```python
from build123d import *

# Parameters (mm, degrees)
SKETCH_R     = 50
PAD_DEPTH    = 3
SKETCH001_R  = 16
POCKET_DEPTH = 3.001
FILLET_R     = 1.2


with BuildPart() as part:
    # Sketch → Pad (new body)
    with BuildSketch(Plane.XY):
        Circle(SKETCH_R)
    extrude(amount=PAD_DEPTH)

    # Sketch001 (on Face3 of Pad) → Pocket (cut, through all)
    with BuildSketch(Plane.XY.offset(3)):
        Circle(SKETCH001_R)
    extrude(amount=-POCKET_DEPTH, mode=Mode.SUBTRACT)

    # Fillet
    fillet_edges = [part.edges().sort_by_distance(p)[0] for p in [
        (-16, 0, 3),
        (16, 0, 1.5),
        (-16, 0, 0),
        (50, 0, 1.5),
        (-50, 0, 0),
        (-50, 0, 3),
    ]]
    fillet(fillet_edges, radius=FILLET_R)


solid = part.part
```
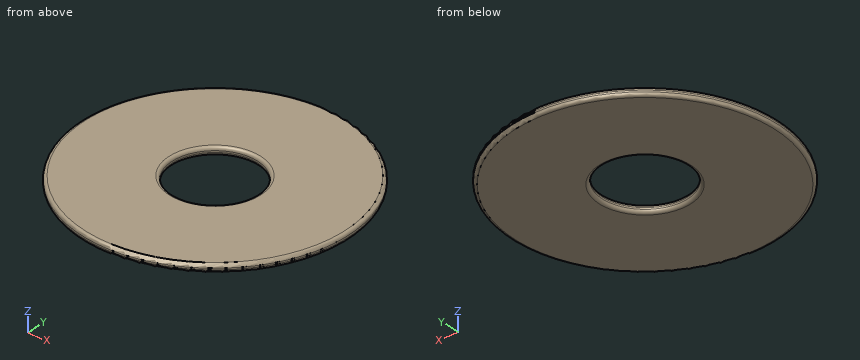
Geometry: final body of the model. Coordinates: model frame, mm. Coordinates: 2 decimals unless noted, no trailing zeros. Loops run counter-clockwise (first coordinate to the right, second up) from the corner with the lowest first, then second, coordinate; pieces in that order, holes last. Notation, with made-up numbers: (3, 67.25) -> (51, 67.25) arc R7 ccw to (51, 76.25) -> close; hole circle Ø3 at (-6.75, 73.5). An arc over 180 degrees is marked (long way). Use a Markdown table: item, result. Add a question column.
(1) Line query: line 1 along Y through (x, z) = (0, 1.6); line 2 along Y through (x, z) = (-3, 2.1); line 3 along X through (y, z) = (11, 0.8). Output: solid intervals per line, ascending.
(2) Section query A-A, the plane x = 0. Return loops of the section in (y, z).
(3) Pin query (flat end, axial travel): pin 1 Ø3 at (x, y) = (20.5, 26.5) entering from -Z; pin 2 Ø1.5 at (x, z) = (-12, 2.5) entering from -Y; pin 3 Ø1 at (x, z) = (32, 1.5) entering from +Y. Return the tip coordinate at first contact, or that it passes through.
(4) Section query C-C, the plane z = 2.4. Return loops of the section in (x, y).
Answer:
| question | item | result |
|---|---|---|
| 1 | line 1 | y = -50 to -16, 16 to 50 |
| 1 | line 2 | y = -49.87 to -15.76, 15.76 to 49.87 |
| 1 | line 3 | x = -48.7 to -11.71, 11.71 to 48.7 |
| 2 | outline | (-50, 1.2) arc R1.2 ccw to (-48.8, 0) -> (-17.2, 0) arc R1.2 ccw to (-16, 1.2) -> (-16, 1.8) arc R1.2 ccw to (-17.2, 3) -> (-48.8, 3) arc R1.2 ccw to (-50, 1.8) -> close; (16, 1.2) arc R1.2 ccw to (17.2, 0) -> (48.8, 0) arc R1.2 ccw to (50, 1.2) -> (50, 1.8) arc R1.2 ccw to (48.8, 3) -> (17.2, 3) arc R1.2 ccw to (16, 1.8) -> close |
| 3 | pin 1 | stops at z = 0 |
| 3 | pin 2 | stops at y = -48.66 |
| 3 | pin 3 | stops at y = 38.83 |
| 4 | outline | circle Ø99.68 at (0, 0); hole circle Ø32.32 at (0, 0) |
